The model under review builds one solid part; all positions refer to its coordinate system, in mm. A direction names the side the tool comes from. Coordinates: 2 decimals unless noted, no trailing zeros. Loops run counter-clockwise (first coordinate to the right, second up) from the corner with the lowest first, then second, coordinate; pieces in that order, holes last. Notation, with made-up numbers: M 51,49.25 L 91,49.25 A16 ccw 91,78.25 Z; hole C 38,8.25 d3. An arc over 180 degrees is marked long. Use one line per item in the form item = value.
Autodesk Inventor part; units mm, degrees
ref_plane "Work Plane1" through (0, 0, 0) normal (0, 0, 1) x (1, 0, 0)
ref_plane "YZ Plane" through (0, 0, 0) normal (1, 0, 0) x (0, 1, 0)
ref_plane "XZ Plane" through (0, 0, 0) normal (0, 1, 0) x (-1, 0, 0)
sketch "Sketch2" plane through (0, 0, 0) normal (0, 0, 1) x (1, 0, 0)
  line L0 (-4, 0) -> (4, 0)
  line L1 (4, 0) -> (4, -12.5)
  line L2 (4, -12.5) -> (-4, -12.5)
  line L3 (-4, -12.5) -> (-4, 0)
  point P0 (0, 0)
  point P1 (0, 0)
  dimension "d8" = 12.5
  dimension "d9" = 8
extrude "Extrusion1" add sketch "Sketch2" along normal mid plane 8
fillet "Fillet1" radius 4 2 edges at (4, -12.5, 0) (-4, -12.5, 0)
sketch "Sketch4" plane through (0, 0, 4) normal (0, 0, 1) x (1, 0, 0)
  line L0 (0, -8.5) -> (0, -4.5) construction
  line L1 (2, -8.5) -> (2, -4.5)
  line L2 (-2, -4.5) -> (-2, -8.5)
  arc A0 (-2, -8.5) -> (2, -8.5) centre (0, -8.5) ccw
  arc A1 (2, -4.5) -> (-2, -4.5) centre (0, -4.5) ccw
  line L3 (4, 0) -> (-4, 0)
  point P0 (0, 0)
  point P1 (0, -6.5)
  point P2 (0, 0)
  dimension "d17" = 4
  dimension "d18" = 2
extrude "Extrusion3" cut sketch "Sketch4" against normal blind 10
sketch "Sketch5" plane through (4, 0, 4) normal (1, 0, 0) x (0, 0, -1)
  line L0 (0, -8.5) -> (0, -8.5)
  line L1 (0, -8.5) -> (8, -8.5)
  line L2 (8, -8.5) -> (8, -8.5)
  line L3 (8, -8.5) -> (0, -8.5)
  line L4 (8, -12.5) -> (0, -12.5)
  line L5 (2, -2.5) -> (6, -2.5)
  line L6 (6, -2.5) -> (6, -12.5)
  line L7 (6, -12.5) -> (2, -12.5)
  line L8 (2, -12.5) -> (2, -2.5)
  line L9 (0, -8.5) -> (0, 0)
  point P0 (4, 0)
  dimension "d22" = 4
  dimension "d23" = 10
  dimension "d24" = 2
extrude "Extrusion4" cut sketch "Sketch5" against normal up to surface (8 mm away)
ref_plane "Work Plane1" through (0, 0, 0) normal (0, 0, 1) x (1, 0, 0)
sketch "Sketch6" plane through (0, 0, 0) normal (0, 0, 1) x (1, 0, 0)
  line L0 (-4, 0) -> (4, 0)
  line L1 (-4, 0) -> (-4.9979, 34.3548)
  arc A0 (0, 39.5) -> (-4.9979, 34.3548) centre (0, 34.5) ccw
  line L2 (0, 39.5) -> (52.1008, 37.9985)
  arc A1 (52.1585, 31.0036) -> (52.1008, 37.9985) centre (52, 34.5) ccw
  line L3 (52.1585, 31.0036) -> (8.2033, 29.0116)
  line L4 (5.343, 26.1684) -> (4, 0)
  arc A2 (0, -2.5) -> (-2, -4.5) centre (0, -4.5) ccw
  arc A3 (2, -4.5) -> (0, -2.5) centre (0, -4.5) ccw
  arc A4 (8.2033, 29.0116) -> (5.343, 26.1684) centre (8.3391, 26.0147) ccw
  point P0 (0, 0)
  point P1 (0, 0)
  dimension "d28" = 5
  dimension "d29" = 39
  dimension "d30" = 52
  dimension "d31" = 3
  dimension "d32" = 3.5
extrude "Extrusion5" add sketch "Sketch6" along normal mid plane 4
sketch "Sketch7" plane through (0, 0, 2) normal (0, 0, 1) x (1, 0, 0)
  arc A0 (52.1585, 31.0036) -> (52.1008, 37.9985) centre (52, 34.5) ccw
  point P0 (0, 0)
hole "Hole1" at (52, 34.5, 2) direction (0, 0, -1) diameter 4 depth 4
sketch "Sketch8" plane through (0, 0, 2) normal (0, 0, 1) x (1, 0, 0)
  arc A0 (0, 39.5) -> (-4.9979, 34.3548) centre (0, 34.5) ccw
  point P0 (0, 0)
hole "Hole2" at (0, 34.5, 2) direction (0, 0, -1) diameter 8 depth 4
sketch "Sketch9" plane through (0, 39.5, 2) normal (0.0288, 0.9996, 0) x (0.9996, -0.0288, 0)
  line L0 (-4.8476, 0) -> (-4.8476, 4)
  line L1 (4.144, 0) -> (-3.856, 0)
  point P0 (1.1378, 2)
  point P1 (0.144, 2)
  point P2 (-4.8476, 2)
  point P3 (0.144, 0)
hole "Hole3" at (0.144, 39.4959, 0) direction (-0.0288, -0.9996, 0) diameter 2.5 depth 12
sketch "Sketch10" plane through (0, 0, -4) normal (0, 0, 1) x (1, 0, 0)
  circle A0 centre (0, -6.592) radius 2
  line L0 (4, 0) -> (-4, 0)
  line L1 (-2, -4.5) -> (-2, -8.5)
  arc A1 (-2, -8.5) -> (2, -8.5) centre (0, -8.5) ccw
  point P0 (0, 0)
  point P1 (0, 0)
  point P2 (-2, -6.5)
  point P3 (0, -10.5)
  dimension "d57" = 4
  dimension "d59" = 3.908
properties part number "10"
1. Insertion check: P1, Ø3, axis at y = 9, z = -0.5, coming from the +X side; P2, Ø1, axis at y = -6.5, z = -3, coming from the -X side; P3, Ø1.6, axis at y = -6.5, z = 3, coming from the +X side; P4, Ø2.5, axis at x = 0, y = -9, coming from the +Z side. Each pin has a flat end and moves straight along its axis. Give the tip position at first contact, or say it passes through.
Response values:
P1 = 4.54
P2 = -4
P3 = 4
P4 = through
2. Machinability: for faces 1 (the face through (0, 0, -3)), 2 (the face through (-2.859, -11.297, -2.986)), 3 (the face through (-2, -6, 3)), 4 (the face through (2, -10, -2)), which of the approach directions +Z, -Z, +X, -X, +Y, -Y give a long, thin tool a straight path to every point of the face, cutting with its end or side? Answer none if there is none.
Response values:
face_1 = -Z, +X, -X, +Y
face_2 = +Z, -Z, -X, -Y
face_3 = +Z, -Z
face_4 = +X, -X, -Y
3. The part is to be moulded in two halves that separate along Y. For faces 5 (the face through (0.322, 29.065, 1.155)), 6 (the face through (0, 0, 3)), 7 (the face through (2.859, -11.297, -3.014)), say which applies: pulls with the +Y half, pulls with the -Y half, needs draft (parallel to the pull), parting line crosses it, or undercut.
Response values:
face_5 = undercut
face_6 = pulls with the +Y half
face_7 = pulls with the -Y half
4. Add section C-C (x = 39). State the section outline as (y, z) points.
Response values:
outline = M 30.41,-2 L 38.38,-2 L 38.38,2 L 30.41,2 Z
5. Wall thickness on line 1 along X through (y, z) = (34.5, -1.1); line 2 along Z through (x, y) = (3.5, -9); line 3 along Y through (x, z) = (52, -0.3): over which ranges is each line inside the solid? List them lowest first. Write a range as from..to.
Response values:
line_1 = -5..-4, 4..50, 54..55.5
line_2 = -4..-2, 2..4
line_3 = 31..32.5, 36.5..38
6. Add section D-D (y = 13.5). State the section outline as (x, z) points, then the cut area to 3 significant figures.
Response values:
outline = M -4.39,-2 L 4.69,-2 L 4.69,2 L -4.39,2 Z
area = 36.3 mm^2
7. Add section B-B (y = 35.5). State the section outline as (x, z) points, then the cut area to 3 significant figures.
Response values:
outline = M -4.9,-2 L -3.87,-2 L -3.87,2 L -4.9,2 Z; M 3.87,-2 L 50.27,-2 L 50.27,2 L 3.87,2 Z; M 53.73,-2 L 55.35,-2 L 55.35,2 L 53.73,2 Z
area = 196 mm^2
